Input: part model. Units: mm. Frame: model coordinates. Coordinates: 2 decimals unless noted, no trailing zeros. Loops run counter-clockwise (first coordinate to the right, second up) from the corner with the lowest first, then second, coordinate; pieces in that order, holes last.
(1) Section C-C, the plane z = 1.6. Return loops of the section in (x, y), then the cut area to 3 significant figures.
(2) Section A-A, the plane x = 24.5. Return loops of the section in (y, z), then the cut area to 4 significant figures.
(3) Section B-B, the plane y = 12.5. Return loops of the section in (x, z), then the cut area to 3 significant figures.
(4) Line query: L1, parallel to Y at x = 24.5, z = 0.6; L2, parallel to Y at x = 24.5, z = 2.8; L3, parallel to X at y = -2.5, z = 2.1. Output: solid intervals per line, ascending.
(5) Section D-D, the plane x = 19.5. Return loops of the section in (y, z).
(6) Contact query for a flat-ended pin moving along its axis: P1, Ø4.5, axis at x = 24.5, y = 12.5, coming from the +Z side. Output: stop coordinate, or through.
```python
from build123d import *

# Parameters (mm, degrees)
F0_W     = 25
F0_H     = 15
F1_DEPTH = 3.5
F2_R     = 1.65
F3_DEPTH = 3.5
F2_R_2   = 2.5
F4_DEPTH = 1


with BuildPart() as f1:
    # F0 (on Top) → F1 (new body)
    with BuildSketch(Plane.XY):
        Polygon((7.5, 20), (-7.5, 20), (-7.5, -20), (7.5, -20), (7.5, 5), align=None)
        with Locations((20, 12.5)):
            Rectangle(F0_W, F0_H)
    extrude(amount=F1_DEPTH)

    # F2 (on face) → F3 (cut, through all)
    with BuildSketch(Plane.XY.offset(3.5)):
        with Locations((0, -12)):
            Circle(F2_R)
        with Locations((24.5, 12.5)):
            Circle(F2_R)
    extrude(amount=-F3_DEPTH, mode=Mode.SUBTRACT)

    # F2 (on face) → F4 (cut)
    with BuildSketch(Plane.XY.offset(3.5)):
        with Locations((0, -12)):
            Circle(F2_R_2)
        with Locations((0, -12)):
            Circle(F2_R, mode=Mode.SUBTRACT)
        with Locations((24.5, 12.5)):
            Circle(F2_R_2)
        with Locations((24.5, 12.5)):
            Circle(F2_R, mode=Mode.SUBTRACT)
    extrude(amount=-F4_DEPTH, mode=Mode.SUBTRACT)


solid = f1.part
```
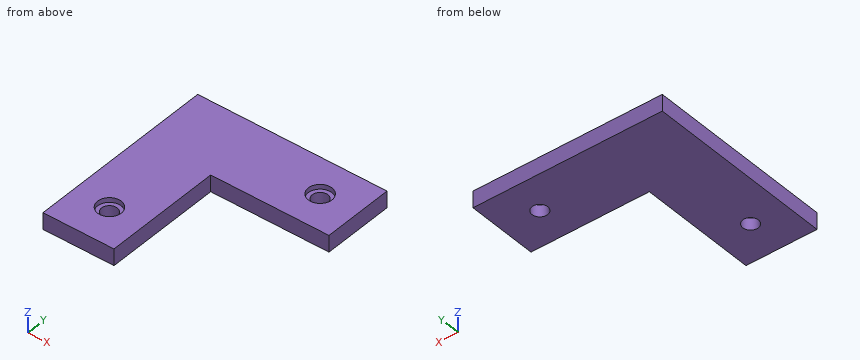
Report:
1. outline: (-7.5, -20) - (7.5, -20) - (7.5, 5) - (32.5, 5) - (32.5, 20) - (-7.5, 20) - close; hole circle Ø3.3 at (0, -12); hole circle Ø3.3 at (24.5, 12.5)
1. area: 958 mm2
2. outline: (5, 0) - (10.85, 0) - (10.85, 2.5) - (10, 2.5) - (10, 3.5) - (5, 3.5) - close; (14.15, 0) - (20, 0) - (20, 3.5) - (15, 3.5) - (15, 2.5) - (14.15, 2.5) - close
2. area: 39.25 mm2
3. outline: (-7.5, 0) - (22.85, 0) - (22.85, 2.5) - (22, 2.5) - (22, 3.5) - (-7.5, 3.5) - close; (26.15, 0) - (32.5, 0) - (32.5, 3.5) - (27, 3.5) - (27, 2.5) - (26.15, 2.5) - close
3. area: 127 mm2
4. L1: y = 5 to 10.85, 14.15 to 20
4. L2: y = 5 to 10, 15 to 20
4. L3: x = -7.5 to 7.5
5. outline: (5, 0) - (20, 0) - (20, 3.5) - (5, 3.5) - close
6. P1: stops at z = 2.5
